Input: part model. Units: mm. Frame: model coordinates. A direction names the side the tool comes from. Round coordinates to 2 decimals unless told otherwise and drop trailing zeros. Write each loop counter-clockwise with the first axis right and the second up, starting at its lowest first coordinate (ties: lowest second). Pieces come first, ordered by that corner, then holes. Notation, with made-up numbers: (46, 44) -> (60, 44) arc R8 ccw to (60, 48) -> close; hole circle Ø7 at (30, 44.5). An arc over 180 degrees is marked (long way). Write item = value, one per line. Start each with the question number.
```python
from build123d import *


with BuildPart() as part:
    # Schizzo1 → Rivoluzione1 (revolve)
    with BuildSketch(Plane.XY, mode=Mode.PRIVATE) as rivoluzione1_sk:
        with BuildLine():
            Line((0, 82.9), (0, 73))
            Line((0, 73), (4.075173742, 73))
            ThreePointArc((4.075173742, 73), (15.761127456, 78.034636074), (25.321314712, 69.6375))
            Line((25.321314712, 69.6375), (30.278685288, 69.6375))
            ThreePointArc((30.278685288, 69.6375), (39.838872544, 78.034636074), (51.524826258, 73))
            Line((51.524826258, 73), (55.6, 73))
            Line((55.6, 73), (55.6, 82.9))
            ThreePointArc((55.6, 82.9), (54.98492424, 84.38492424), (53.5, 85))
            Line((53.5, 85), (2.1, 85))
            ThreePointArc((2.1, 85), (0.61507576, 84.38492424), (0, 82.9))
        make_face()
    revolve(rivoluzione1_sk.sketch.rotate(Axis((27.8, 0, 0), (-1, 0, 0)), 270), axis=Axis((27.8, 0, 0), (-1, 0, 0)))


solid = part.part
```
1. Section C-C (x = 12). Output: boundary loops of the cut face in (y, z).
2. Reachability of faces 1 (the flat face through (55.6, -73.3, 0.4)), 2 (the cylindrical face through (2.066, -71.264, -15.825)), 3 (the cylindrical face through (53.591, -71.264, -15.825)) from +Z, -Z, +X, -X, +Y, -Y: full face, straight path, thin tool, end or side. Return the list, or none.
3. Line query: line 1 along Y through (x, z) = (26.55, 0); line 2 along X through (y, z) = (1, 73.5); line 3 along X through (y, z) = (-74, 3.5). Output: solid intervals per line, ascending.
4. Mould query, pull axis Y, two halves, no side actions, for faces 4 (the cylindrical face through (27.44, -51.721, -67.453)), 5 (the cylindrical face through (27.83, 20.92, 66.42)), 6 (the flat face through (0, -73.3, -0.4)). Classes: pulls with the +Y half, pulls with the -Y half, needs draft (parallel to the pull), parting line crosses it, or undercut.
5. Section D-D (x = 32.5). Output: boundary loops of the cut face in (y, z), then the cut area to 3 significant figures.
6. Pin query (flat end, axial travel): P1, Ø12, axis at x = 32.5, z = 60.5, coming from the -Y side; P2, Ø3, axis at x = 37.5, z = 37, coming from the -Y side; P3, Ø8, axis at x = 45, z = 67.5, coming from the -Y side. Return the tip coordinate at first contact, or that it passes through.
7. Section A-A (z = 0). Output: boundary loops of the cut face in (x, y) (1 decimal).
Check sheet entries:
q1.outline = circle Ø170 at (0, 0); hole circle Ø156.06 at (0, 0)
q2.face_1 = +Z, -Z, +X, +Y, -Y
q2.face_2 = -X
q2.face_3 = +X
q3.line_1 = -85 to -69.64, 69.64 to 85
q3.line_2 = 0 to 4.44, 23.36 to 32.24, 51.16 to 55.6
q3.line_3 = 0 to 4.91, 22.89 to 32.71, 50.69 to 55.6
q4.face_4 = parting line crosses it
q4.face_5 = undercut
q4.face_6 = needs draft
q5.outline = circle Ø170 at (0, 0); hole circle Ø147.66 at (0, 0)
q5.area = 5,570 mm2
q6.P1 = -65.23
q6.P2 = -77.23
q6.P3 = -56.5
q7.outline = (0, -82.9) arc R2.1 ccw to (2.1, -85) -> (53.5, -85) arc R2.1 ccw to (55.6, -82.9) -> (55.6, -73) -> (51.5, -73) arc R11.9 cw to (30.3, -69.6) -> (25.3, -69.6) arc R11.9 cw to (4.1, -73) -> (0, -73) -> close; (0, 73) -> (4.1, 73) arc R11.9 cw to (25.3, 69.6) -> (30.3, 69.6) arc R11.9 cw to (51.5, 73) -> (55.6, 73) -> (55.6, 82.9) arc R2.1 ccw to (53.5, 85) -> (2.1, 85) arc R2.1 ccw to (0, 82.9) -> close
